```python
from build123d import *

# Parameters (mm, degrees)
F0_R     = 5.5
F0_R_2   = 5
F1_DEPTH = 5
F2_DEPTH = 2


with BuildPart() as f1:
    # F0 (on Front) → F1 (new body)
    with BuildSketch(Plane.XZ):
        with BuildLine():
            Line((40.64, 10), (0, 10))
            ThreePointArc((0, 10), (-10, 0), (0, -10))
            Line((0, -10), (40.64, -10))
            ThreePointArc((40.64, -10), (50.64, 0), (40.64, 10))
        make_face()
        Circle(F0_R, mode=Mode.SUBTRACT)
        with Locations((40.64, 0)):
            Circle(F0_R, mode=Mode.SUBTRACT)
        Circle(F0_R)
        Circle(F0_R_2, mode=Mode.SUBTRACT)
        with Locations((40.64, 0)):
            Circle(F0_R)
        with Locations((40.64, 0)):
            Circle(F0_R_2, mode=Mode.SUBTRACT)
    extrude(amount=F1_DEPTH)

    # F0 (on Front) → F2 (cut)
    with BuildSketch(Plane.XZ):
        with Locations((40.64, 0)):
            Circle(F0_R)
        with Locations((40.64, 0)):
            Circle(F0_R_2, mode=Mode.SUBTRACT)
        Circle(F0_R)
        Circle(F0_R_2, mode=Mode.SUBTRACT)
    extrude(amount=F2_DEPTH, mode=Mode.SUBTRACT)


solid = f1.part
```
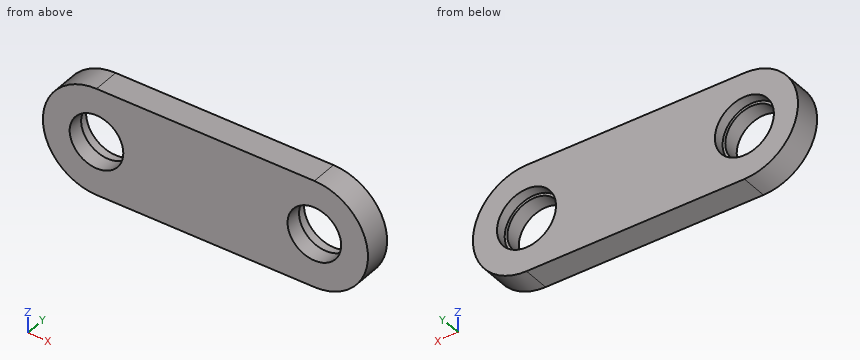
Geometry: final body of the model. Coordinates: model frame, mm. Coordinates: 2 decimals unless noted, no trailing zeros. Order: outer loops, then holes, each group sorted by start corner. A loop starts at its lowest first (then second) coordinate and runs counter-clockwise, first axis right, second up. Notation, with made-up numbers: (11, 8) -> (45, 8) arc R19 cw to (45, 23) -> close; hole circle Ø2 at (25, 13). An arc over 180 degrees is marked (long way). Answer in a Markdown table with one row per item.
Item 1: Section A-A on z = 0. Output: boundary loops of the cut face in (x, y), plus the area to 3 significant figures.
Return value:
| item | result |
|---|---|
| outline | (-10, -5) -> (-5, -5) -> (-5, -2) -> (-5.5, -2) -> (-5.5, 0) -> (-10, 0) -> close; (5, -5) -> (35.64, -5) -> (35.64, -2) -> (35.14, -2) -> (35.14, 0) -> (5.5, 0) -> (5.5, -2) -> (5, -2) -> close; (45.64, -5) -> (50.64, -5) -> (50.64, 0) -> (46.14, 0) -> (46.14, -2) -> (45.64, -2) -> close |
| area | 199 mm² |
Item 2: Ray query, L1, parallel to Z at x = 40.64, y = -3.9; L2, parallel to X at y = -3.95, z = -3.5; L3, parallel to Z at x = 0, y = -0.7. Return the intervals inside material, ascending.
Return value:
| item | result |
|---|---|
| L1 | z = -10 to -5, 5 to 10 |
| L2 | x = -9.37 to -3.57, 3.57 to 37.07, 44.21 to 50.01 |
| L3 | z = -10 to -5.5, 5.5 to 10 |
Item 3: Section D-D on z = -3. Output: boundary loops of the cut face in (x, y), plus the area to 3 significant figures.
Return value:
| item | result |
|---|---|
| outline | (-9.54, -5) -> (-4, -5) -> (-4, -2) -> (-4.61, -2) -> (-4.61, 0) -> (-9.54, 0) -> close; (4, -5) -> (36.64, -5) -> (36.64, -2) -> (36.03, -2) -> (36.03, 0) -> (4.61, 0) -> (4.61, -2) -> (4, -2) -> close; (44.64, -5) -> (50.18, -5) -> (50.18, 0) -> (45.25, 0) -> (45.25, -2) -> (44.64, -2) -> close |
| area | 214 mm² |
Item 4: Section C-C on z = 8. Output: boundary loops of the cut face in (x, y).
Return value:
| item | result |
|---|---|
| outline | (-6, -5) -> (46.64, -5) -> (46.64, 0) -> (-6, 0) -> close |
Item 5: Section B-B on x = -4. Output: boundary loops of the cut face in (y, z).
Return value:
| item | result |
|---|---|
| outline | (-5, -9.17) -> (0, -9.17) -> (0, -3.77) -> (-2, -3.77) -> (-2, -3) -> (-5, -3) -> close; (-5, 3) -> (-2, 3) -> (-2, 3.77) -> (0, 3.77) -> (0, 9.17) -> (-5, 9.17) -> close |
Item 6: Contact query for flat-ended pins moving along their axis: P1, Ø1.5, axis at y = -3, z = -0.5, coming from the +X side; P2, Ø1, axis at y = -4, z = -6, coming from the -X side; P3, Ø2, axis at x = 43, y = -2, coming from the -Z side. Output: stop coordinate, or through.
Return value:
| item | result |
|---|---|
| P1 | stops at x = 50.64 |
| P2 | stops at x = -8.35 |
| P3 | stops at z = -9.91 |
